Build history of the part. All positions in model axes, mm. A direction names the side the tool comes from. Give positions to 0.01 mm unless a question says otherwise; leave off trailing zeros. Write each loop counter-clockwise with the first axis right and the second up, starting at its lowest first coordinate (ties: lowest second). Pieces come first, ordered by that corner, then holes.
from build123d import *

# Parameters (mm, degrees)
EXTRUDE_1_DEPTH = 1.5
EXTRUDE_2_DEPTH = 3
FILLET_1_R      = 1.5


with BuildPart() as part:
    # 草圖1 → 擠出1 (new body)
    with BuildSketch(Plane.XY):
        Polygon((-16, 0), (0, 16), (0, 111), (-16, 111), (-16, 97.073509127), (-98.206395117, 0), align=None)
    extrude(amount=EXTRUDE_1_DEPTH)

    # 草圖2 → 擠出2 (add)
    with BuildSketch(Plane.XY):
        Polygon((-110, 0), (-98.206395117, 0), (-16, 97.073509127), (-16, 111), align=None)
    extrude(amount=EXTRUDE_2_DEPTH)

    # 圓角1
    fillet_1_edges = [part.edges().sort_by_distance(p)[0] for p in [
        (-63, 55.5, 0),
        (-63, 55.5, 3),
    ]]
    fillet(fillet_1_edges, radius=FILLET_1_R - 0.0001)  # a hair under: the kernel refuses the full size


solid = part.part
1. Drop flat-ended pins along their axis: pin 1 (1.2 mm diameter, centred on y = 105.5, z = 2.5, fed in from +X); pin 2 (10 mm diameter, centred on x = -17, y = 25, fed in from +Z). Give the stop position or say it passes through.
2. Saw through at A-A on x = -8. Give the cut face in (y, z).
3. 3-axis set-ups, long thin cutter, end or side, ignore diameter. For faces 1 (the face through (-28, 44, 1.5)), 2 (the face through (-59, 51, 3)): which of +Z, -Z, +X, -X, +Y, -Y reach the whole face in a straight line?
4. Saw through at B-B on z = 2. Give the cut face in (x, y), plus the area to 3 significant figures.
5. Drill centre lines: line 1 along Z through (x, y) = (-14.5, 85.5); line 2 along Y through (x, z) = (-14.5, 1.2); line 3 along Z through (x, y) = (-38, 83). Where is each one in solid material? Low to high.
Outcome:
1. pin 1: stops at x = -16
1. pin 2: stops at z = 1.5
2. outline: (8, 0) - (111, 0) - (111, 1.5) - (8, 1.5) - close
3. face 1: +Z, +X, -Y
3. face 2: +Z, +X, -X, +Y, -Y
4. outline: (-109.89, 0) - (-98.21, 0) - (-16, 97.07) - (-16, 110.87) - close
4. area: 1,210 mm2
5. line 1: z = 0 to 1.5
5. line 2: y = 1.5 to 111
5. line 3: z = 0.01 to 2.99
